For this review, take the finished solid that the model builds, in its own axes (mm). Face numbers are marked on the shaded views. A direction names the side the tool comes from. Give positions to 0.01 mm unless a question says otherwise; leave off trailing zeros. Write each loop counter-clockwise with the first axis right and the second up, starting at its lowest first coordinate (ties: lowest second). Pieces come first, ordered by that corner, then holes.
Q1. Machinability: for the marked faces 4 and 5, which of the approach directions +Z, -Z, +X, -X, +Y, -Y give a long, thin tool a straight path to every point of the face, cutting with its end or side? Answer none if there is none.
Q2. For line 1 (Z direction, x = 16, y = 33); line 2 (Z direction, x = 22.5, y = 22.5); line 3 (Y direction, x = 46.5, z = 13), list the stretches that pass through material, from the lowest coordinate up.
Q3. We need section D-D (x = 16.5). Write out the cut boundary in (y, z), then the cut area to 3 significant figures.
Q4. We need section C-C (z = 15). Write out the cut boundary in (x, y), then the cut area to 3 significant figures.
Q5. We need section B-B (y = 39.5). Write out the cut boundary in (x, z) (3 decimals), then the cut area to 3 significant figures.
Q6. Insertion check: P1, Ø1, axis at y = 36.5, z = 39, coming from the +X side; P2, Ø12, axis at x = 13.5, z = 36.5, coming from the +Y side. Each pin has a flat end and moves straight along its axis. Give the tip position at first contact, or say it passes through.
Q7. We need section A-A (x = 44). Write out the cut boundary in (y, z), then the cut area to 3 significant figures.
Q8. Mouldability with a two-part tool opening along Z and no side actions: class the marked faces 1, 2 and 3 as released by +Z, released by -Z, zero draft, split by the parting line, or undercut.
```python
from build123d import *

# Parameters (mm, degrees)
EXTRUDE1_DEPTH     = 70
CUT_EXTRUDE1_DEPTH = 51


with BuildPart() as part:
    # Sketch1 → Extrude1 (new body)
    with BuildSketch(Plane.XY):
        Polygon((30, 65), (0, 25), (0, 0), (50, 0), (50, 65), align=None)
    extrude(amount=EXTRUDE1_DEPTH)

    # Sketch2 → Cut-Extrude1 (cut, through all)
    with BuildSketch(Plane(origin=(50, 0, 0), x_dir=(0, 0, -1), z_dir=(1, 0, 0))):
        Polygon((-70, 0), (-70, 65), (-40, 65), align=None)
        Polygon((-32.5, 48.97114317), (-10, 10), (-55, 10), align=None)
    extrude(amount=-CUT_EXTRUDE1_DEPTH, mode=Mode.SUBTRACT)


solid = part.part
```
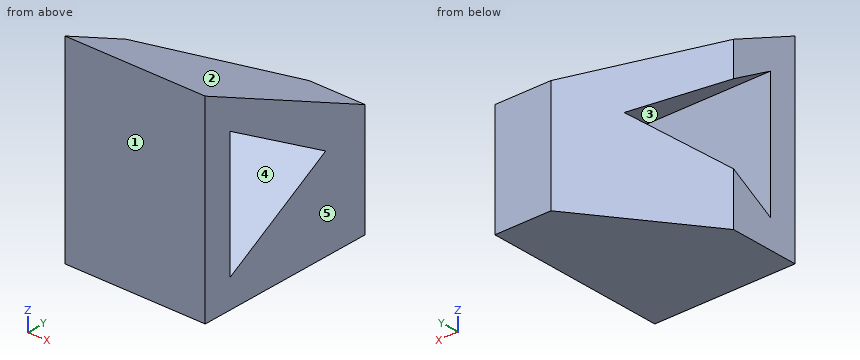
Computed:
1. face 4: +X, -X
1. face 5: +Z, -Z, +X, +Y, -Y
2. line 1: z = 0 to 23.28, 41.72 to 54.77
2. line 2: z = 0 to 17.22, 47.78 to 59.62
2. line 3: y = 0 to 10, 15.2 to 65
3. outline: (0, 0) - (47, 0) - (47, 31.36) - (10, 10) - (10, 55) - (47, 33.64) - (47, 48.31) - (0, 70) - close
3. area: 1,910 mm2
4. outline: (0, 0) - (50, 0) - (50, 10) - (0, 10) - close; (0, 18.66) - (50, 18.66) - (50, 65) - (30, 65) - (0, 25) - close
4. area: 2,220 mm2
5. outline: (10.875, 0) - (50, 0) - (50, 27.032) - (10.875, 27.032) - close; (10.875, 37.968) - (50, 37.968) - (50, 51.769) - (10.875, 51.769) - close
5. area: 1,600 mm2
6. P1: passes through
6. P2: stops at y = 51
7. outline: (0, 0) - (65, 0) - (65, 40) - (0, 70) - close; hole (10, 10) - (48.97, 32.5) - (10, 55) - close
7. area: 2,700 mm2
8. face 1: zero draft
8. face 2: released by +Z
8. face 3: undercut
